Can you work these out from the model? Positions are in its coordinate system, mm. A direction names the side the tool comes from. Round coordinates to 2 decimals unless told otherwise and drop trailing zeros. Loops run counter-clockwise (first coordinate to the right, second up) from the corner with the lowest first, then second, coordinate; pieces in that order, holes last. Notation, with made-up numbers: (65.5, 80.25) -> (95.5, 80.25) arc R23 ccw to (95.5, 116.25) -> close; hole circle Ø2 at (75.25, 71.5). An arc over 180 degrees is marked (long way). Use a Markdown table: item, result.
from build123d import *

# Parameters (mm, degrees)
CROQUIS1_W              = 50
CROQUIS1_H              = 50
CROQUIS1_W_2            = 44
CROQUIS1_H_2            = 44
SALIENTE_EXTRUIR1_DEPTH = 750


with BuildPart() as part:
    # Croquis1 → Saliente-Extruir1 (new, symmetric)
    with BuildSketch(Plane.XY):
        Rectangle(CROQUIS1_W, CROQUIS1_H)
        Rectangle(CROQUIS1_W_2, CROQUIS1_H_2, mode=Mode.SUBTRACT)
    extrude(amount=SALIENTE_EXTRUIR1_DEPTH, both=True)


solid = part.part
1. I want a section at B-B (z = 267.5). Please give me the cut outline in (x, y).
Answer sheet:
| item | result |
|---|---|
| outline | (-25, -25) -> (25, -25) -> (25, 25) -> (-25, 25) -> close; hole (-22, -22) -> (22, -22) -> (22, 22) -> (-22, 22) -> close |
2. I need wall thicknesses on line 1 (Y direction, x = 0.5, z = -338). Which ranges of the line are inside material? Lowest first, please.
Answer sheet:
| item | result |
|---|---|
| line 1 | y = -25 to -22, 22 to 25 |
3. If we mould it in two halves opening along X, with no side actions, what happens to faces 1 (the flat face through (0, -22, 10)), 2 (the flat face through (22, 0, 10)), 3 (the flat face through (25, 0, 10)), 4 (the flat face through (-22.3, 0.1, -750))? For each: +X half, -X half, draft (parallel to the pull), parting line (faces both ways), or undercut.
Answer sheet:
| item | result |
|---|---|
| face 1 | undercut |
| face 2 | undercut |
| face 3 | +X half |
| face 4 | draft |
4. Will this pin go through, and if not, where does the flat tip stop? pin 1 Ø5 at (x, y) = (-11, 18) entering from -Z.
Answer sheet:
| item | result |
|---|---|
| pin 1 | passes through |
5. I want a section at A-A (y = -3.5). Please give me the cut outline in (x, z), plus the area to 3 significant figures.
Answer sheet:
| item | result |
|---|---|
| outline | (-25, -750) -> (-22, -750) -> (-22, 750) -> (-25, 750) -> close; (22, -750) -> (25, -750) -> (25, 750) -> (22, 750) -> close |
| area | 9,000 mm² |
6. Which directions (+Z, -Z, +X, -X, +Y, -Y) give clear straight access to the entire face, cutting with the end or side of a thin tool? Please do faces 5 (the flat face through (0, 22, 10)), 6 (the flat face through (0, -25, 10)).
Answer sheet:
| item | result |
|---|---|
| face 5 | +Z, -Z |
| face 6 | +Z, -Z, +X, -X, -Y |
